Here's the drawing with two shaded views (mm, measured from the low corner). I have some questions. Give positions to 0.01 mm unless a question says otherwise; leave off trailing zeros. Loops run counter-clockwise (first coordinate to the right, second up) from the corner with the lowest first, then second, coordinate; pieces in that order, holes last. Notation, with made-up numbers: (74.25, 70.5) - (102.25, 70.5) arc R14 cw to (102.25, 84.5) - close; hole circle Ø11 at (83, 83). An arc over 180 degrees is marked (long way). Write each question's results on one line, items separated by ' | '. Start each with the question number.
1) I want a section at C-C, the plane z = 89. Write out the boundary of the cut face in (x, y).
2) If I drill on probe 1 along X at (y, z) = (0.3, 149); probe 2 along X at (y, z) = (2.55, 16.5); probe 3 along X at (y, z) = (0.9, 51), over which ranges is the centre line in solid material (lowest first)? Write a range as [from, to].
3) I'm going to push flat-ended pins straight in: pin 1 (1 mm diameter, centred on y = 1.5, z = 131, fed in from -X); pin 2 (4.5 mm diameter, centred on x = 241.61, z = 59.39, fed in from +Y); pin 3 (3 mm diameter, centred on x = 241.61, z = 80.61, fed in from -Y); pin 4 (1.5 mm diameter, centred on x = 20.5, y = 2, fed in from +Z). Where does each tip first touch, or does it pass through?
4) I want a section at B-B, the plane x = 20. Write out the boundary of the cut face in (y, z), and give its area (3 significant figures).
5) I want a section at A-A, the plane y = 0.7. Count the separate pieces of the cut face and the enclosed holes in it, and give its area (3 significant figures).
6) I want a section at D-D, the plane z = 132. Write out the boundary of the cut face in (x, y), and give its area (3 significant figures).
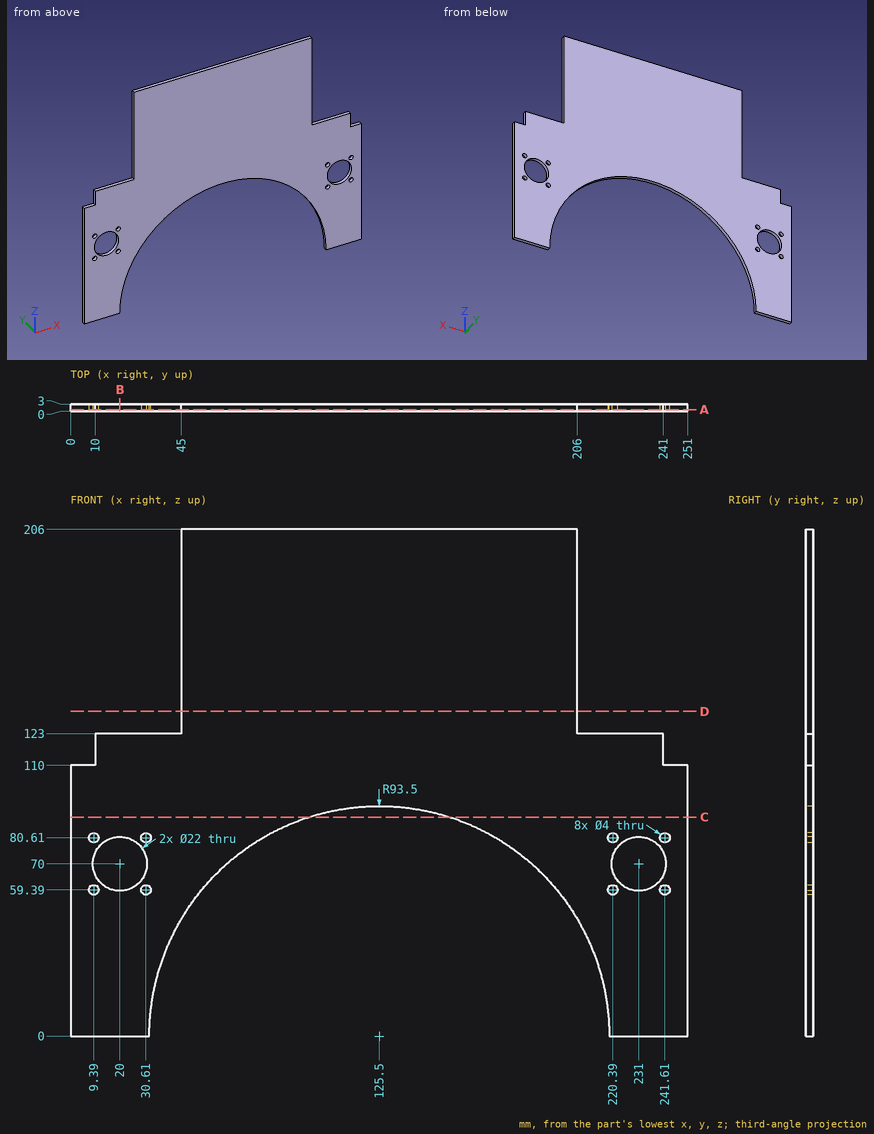
Answers:
1) outline: (0, 0) - (96.84, 0) - (96.84, 3) - (0, 3) - close; (154.16, 0) - (251, 0) - (251, 3) - (154.16, 3) - close
2) probe 1: x = [45, 206] | probe 2: x = [0, 33.47], [217.53, 251] | probe 3: x = [0, 47.13], [203.87, 251]
3) pin 1: stops at x = 45 | pin 2: stops at y = 3 | pin 3: passes through | pin 4: stops at z = 123
4) outline: (0, 0) - (3, 0) - (3, 59) - (0, 59) - close; (0, 81) - (3, 81) - (3, 123) - (0, 123) - close | area: 303 mm2
5) separate pieces: 1 | enclosed holes: 10 | area: 29,400 mm2
6) outline: (45, 0) - (206, 0) - (206, 3) - (45, 3) - close | area: 483 mm2
